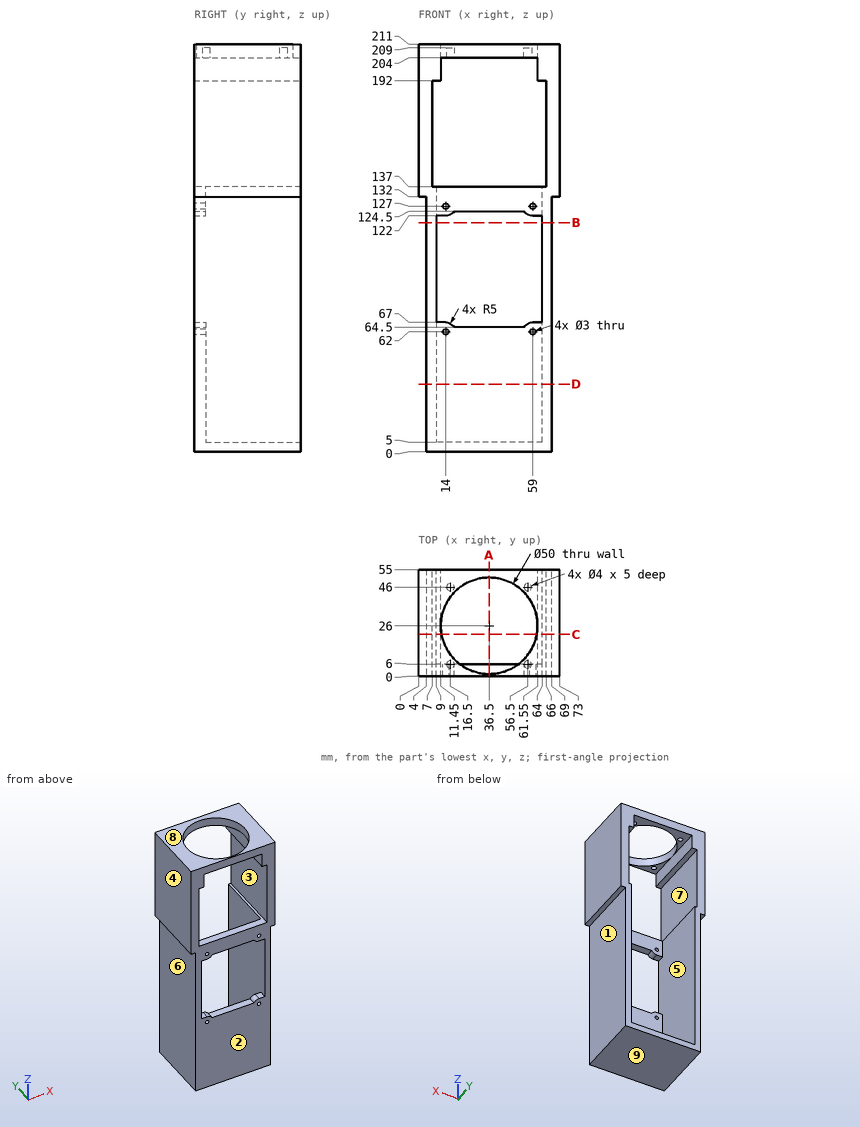
Design review of the part shown in the three views and the two pictorial views. Dimensions are in mm from the part's minimum x, y and z. A direction names the side the tool comes from. Give positions to 0.01 mm unless a question says otherwise; leave off trailing zeros. Loops run counter-clockwise (first coordinate to the right, second up) from the corner with the lowest first, then second, coordinate; pieces in that order, holes last. Notation, with made-up numbers: M 66,33 L 120,33 A9 ccw 120,49 Z; hole C 48.5,84.5 d3. An arc over 180 degrees is marked long. Put each result on its own line as item: value. Start each with the question number.
(1) Add section C-C, the plane y = 21.5. Write out the cut boundary in (x, z).
(2) Wall thickness on L1, parallel to Z at x = 14, y = 1.55; L2, parallel to X at y = 41, z = 73; L3, parallel to Z at x = 7.5, y = 18: over which ranges is each line inside the solid? List them lowest first.
(3) Machinability: for the marked faces 1, 2, 3, 4 and 5, which of the approach directions +Z, -Z, +X, -X, +Y, -Y give a long, thin tool a straight path to every point of the face, cutting with its end or side? Answer none if there is none.
(4) Add section A-A, the plane x = 36.5. Write out the cut boundary in (y, z), then the cut area to 3 significant figures.
(5) Add section B-B, the plane z = 118.5. Write out the cut boundary in (x, y).
(6) For pin 1 (1 mm diameter, centred on y = 48, z = 121, fed in from +X); pin 2 (2 mm diameter, centred on x = 2, y = 22, fed in from -Z); pin 3 (1.8 mm diameter, centred on x = 42, y = 4, fed in from +Z), all flat-tipped, find the tip position at first contact; note any pin that passes through.
(7) Add section D-D, the plane z = 35. Write out the cut boundary in (x, y).
(8) The part is to be moulded in two halves that separate along Z. For the marked faces 6, 7, 8 and 9, say which applies: +Z half, -Z half, draft (parallel to the pull), parting line (faces both ways), or undercut.
Result:
1. outline: M 0,132 L 4,132 L 4,0 L 69,0 L 69,132 L 73,132 L 73,211 L 61.09,211 L 61.09,204 L 61.55,204 L 61.55,192 L 66,192 L 66,137 L 64,137 L 64,5 L 9,5 L 9,137 L 7,137 L 7,192 L 11.45,192 L 11.45,204 L 11.91,204 L 11.91,211 L 0,211 Z
2. L1: z = 0 to 60.5, 63.5 to 67, 122 to 125.5, 128.5 to 137, 204 to 211
2. L2: x = 4 to 9, 64 to 69
2. L3: z = 0 to 137, 192 to 211
3. face 1: -Z, +X, +Y, -Y
3. face 2: +Z, -Z, +X, -X, -Y
3. face 3: +Y, -Y
3. face 4: +Z, -Z, -X, +Y, -Y
3. face 5: +Y
4. outline: M 0,0 L 55,0 L 55,5 L 6,5 L 6,64.5 L 0,64.5 Z; M 0,124.5 L 6,124.5 L 6,137 L 0,137 Z; M 0,204 L 1,204 L 1,211 L 0,211 Z; M 51,204 L 55,204 L 55,211 L 51,211 Z
4. area: 742 mm^2
5. outline: M 4,0 L 9,0 L 9,55 L 4,55 Z; M 64,0 L 69,0 L 69,55 L 64,55 Z
6. pin 1: stops at x = 69
6. pin 2: stops at z = 132
6. pin 3: stops at z = 137
7. outline: M 4,0 L 69,0 L 69,55 L 64,55 L 64,6 L 9,6 L 9,55 L 4,55 Z
8. face 6: draft
8. face 7: undercut
8. face 8: +Z half
8. face 9: -Z half
